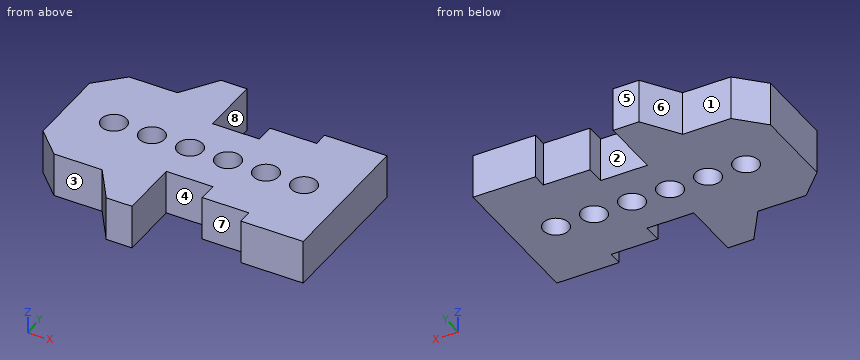
from build123d import *

# Parameters (mm, degrees)
BOSS_EXTRUDE1_DEPTH = 22.225


with BuildPart() as part:
    # Sketch4 → Boss-Extrude1 (new body)
    with BuildSketch(Plane.XY):
        with BuildLine():
            Line((-49.139399536, 0.154397006), (-66.665399536, 0.154397006))
            Line((-66.665399536, 0.154397006), (-66.665399536, -20.419602994))
            Line((-66.665399536, -20.419602994), (-53.965399536, -33.119602994))
            Line((-53.965399536, -33.119602994), (-29.835399536, -33.119602994))
            Line((-29.835399536, -33.119602994), (-17.897399536, -50.645602994))
            Line((-17.897399536, -50.645602994), (-4.943399536, -50.645602994))
            Line((-4.943399536, -50.645602994), (-4.943399536, -20.419602994))
            Line((-4.943399536, -20.419602994), (18.424600464, -20.419602994))
            Line((18.424600464, -20.419602994), (18.424600464, -29.817602994))
            Line((18.424600464, -29.817602994), (41.792600464, -29.817602994))
            Line((41.792600464, -29.817602994), (41.792600464, -36.929602994))
            Line((41.792600464, -36.929602994), (73.034600464, -36.929602994))
            Line((73.034600464, -36.929602994), (73.034600464, 0.154397006))
            Line((73.034600464, 0.154397006), (58.810600464, 0.154397006))
            ThreePointArc((58.810600464, 0.154397006), (52.460600464, -6.195602994), (46.110600464, 0.154397006))
            Line((46.110600464, 0.154397006), (39.760600464, 0.154397006))
            ThreePointArc((39.760600464, 0.154397006), (33.410600464, -6.195602994), (27.060600464, 0.154397006))
            Line((27.060600464, 0.154397006), (20.710600464, 0.154397006))
            ThreePointArc((20.710600464, 0.154397006), (14.360600464, -6.195602994), (8.010600464, 0.154397006))
            Line((8.010600464, 0.154397006), (1.660600464, 0.154397006))
            ThreePointArc((1.660600464, 0.154397006), (-4.689399536, -6.195602994), (-11.039399536, 0.154397006))
            Line((-11.039399536, 0.154397006), (-17.389399536, 0.154397006))
            ThreePointArc((-17.389399536, 0.154397006), (-23.739399536, -6.195602994), (-30.089399536, 0.154397006))
            Line((-30.089399536, 0.154397006), (-36.439399536, 0.154397006))
            ThreePointArc((-36.439399536, 0.154397006), (-42.789399536, -6.195602994), (-49.139399536, 0.154397006))
        make_face()
        with BuildLine():
            Line((-53.965399536, 33.428397006), (-66.665399536, 20.728397006))
            Line((-66.665399536, 20.728397006), (-66.665399536, 0.154397006))
            Line((-66.665399536, 0.154397006), (-49.139399536, 0.154397006))
            ThreePointArc((-49.139399536, 0.154397006), (-42.789399536, 6.504397006), (-36.439399536, 0.154397006))
            Line((-36.439399536, 0.154397006), (-30.089399536, 0.154397006))
            ThreePointArc((-30.089399536, 0.154397006), (-23.739399536, 6.504397006), (-17.389399536, 0.154397006))
            Line((-17.389399536, 0.154397006), (-11.039399536, 0.154397006))
            ThreePointArc((-11.039399536, 0.154397006), (-4.689399536, 6.504397006), (1.660600464, 0.154397006))
            Line((1.660600464, 0.154397006), (8.010600464, 0.154397006))
            ThreePointArc((8.010600464, 0.154397006), (14.360600464, 6.504397006), (20.710600464, 0.154397006))
            Line((20.710600464, 0.154397006), (27.060600464, 0.154397006))
            ThreePointArc((27.060600464, 0.154397006), (33.410600464, 6.504397006), (39.760600464, 0.154397006))
            Line((39.760600464, 0.154397006), (46.110600464, 0.154397006))
            ThreePointArc((46.110600464, 0.154397006), (52.460600464, 6.504397006), (58.810600464, 0.154397006))
            Line((58.810600464, 0.154397006), (73.034600464, 0.154397006))
            Line((73.034600464, 0.154397006), (73.034600464, 37.238397006))
            Line((73.034600464, 37.238397006), (41.792600464, 37.238397006))
            Line((41.792600464, 37.238397006), (41.792600464, 30.126397006))
            Line((41.792600464, 30.126397006), (18.424600464, 30.126397006))
            Line((18.424600464, 30.126397006), (18.424600464, 20.728397006))
            Line((18.424600464, 20.728397006), (-4.943399536, 20.728397006))
            Line((-4.943399536, 20.728397006), (-4.943399536, 50.954397006))
            Line((-4.943399536, 50.954397006), (-17.897399536, 50.954397006))
            Line((-17.897399536, 50.954397006), (-29.835399536, 33.428397006))
            Line((-29.835399536, 33.428397006), (-53.965399536, 33.428397006))
        make_face()
    extrude(amount=BOSS_EXTRUDE1_DEPTH)


solid = part.part
Build history of the part. All positions in model axes, mm. Face numbers are marked on the shaded views. A direction names the side the tool comes from. Round coordinates to 2 decimals unless told otherwise and drop trailing zeros. Write each loop counter-clockwise with the first axis right and the second up, starting at its lowest first coordinate (ties: lowest second). Pieces come first, ordered by that corner, then holes. Notation, with made-up numbers: M 73.5,73.25 L 125.5,73.25 A27 cw 125.5,89.25 Z; hole C 85.25,-23.5 d6. An arc over 180 degrees is marked long. Answer as a JSON object with one key per item and string values. Group by question number.
(1) Drill centre lines: L1, parallel to Y at x = 63, z = 5; L2, parallel to Y at x = 3.5, z = 13.5; L3, parallel to X at y = 22, z = 3.5. Where is each one in solid material? Low to high.
(2) Mould opens along X. For the marked faces 5, 6, 7 and 8 say: pulls with the +X half, pulls with the -X half, needs draft (parallel to the pull), parting line crosses it, or undercut.
(3) Cut at A-A (x = -2). Give the cut face in (y, z) (3 decimals).
(4) Cut at C-C (x = 44). Give the cut face in (y, z) (3 decimals), and give its area (3 significant figures).
(5) Flat gauge pins, fed straight in: pin 1 (6.5 mm diameter, centred on x = 3.5, z = 15, fed in from -Y); pin 2 (6.5 mm diameter, centred on x = -42.5, z = 11, fed in from +Y); pin 3 (6.5 mm diameter, centred on x = 28, z = 9, fed in from +Y). Where does each tip first touch, or does it go through?
(6) Cut at D-D (y = -42). Give the cut face in (x, z) (3 decimals).
(7) Which spindle directions (+Z, -Z, +X, -X, +Y, -Y) get a long thin tool onto all of the face, cutting with end or side? Do the marked faces 1, 2, 3 and 4. Say none if no direction does.
(8) Cut at B-B (z = 12.5). Give the cut face in (x, y).
Responses:
{
 "1": {"L1": "y = -36.93 to 37.24", "L2": "y = -20.42 to 20.73", "L3": "x = -65.39 to -4.94, 18.42 to 73.03"},
 "2": {"face 5": "needs draft", "face 6": "pulls with the -X half", "face 7": "undercut", "face 8": "undercut"},
 "3": {"outline": "M -20.42,0 L -5.598,0 L -5.598,22.225 L -20.42,22.225 Z; M 5.907,0 L 20.728,0 L 20.728,22.225 L 5.907,22.225 Z"},
 "4": {"outline": "M -36.93,0 L 37.238,0 L 37.238,22.225 L -36.93,22.225 Z", "area": "1,650 mm2"},
 "5": {"pin 1": "stops at y = -20.42", "pin 2": "stops at y = 33.43", "pin 3": "stops at y = 30.13"},
 "6": {"outline": "M -23.786,0 L -4.943,0 L -4.943,22.225 L -23.786,22.225 Z"},
 "7": {"face 1": "+Z, -Z, -X, +Y", "face 2": "+Z, -Z, +Y", "face 3": "+Z, -Z, -X, -Y", "face 4": "+Z, -Z, -Y"},
 "8": {"outline": "M -66.67,-20.42 L -53.97,-33.12 L -29.84,-33.12 L -17.9,-50.65 L -4.94,-50.65 L -4.94,-20.42 L 18.42,-20.42 L 18.42,-29.82 L 41.79,-29.82 L 41.79,-36.93 L 73.03,-36.93 L 73.03,37.24 L 41.79,37.24 L 41.79,30.13 L 18.42,30.13 L 18.42,20.73 L -4.94,20.73 L -4.94,50.95 L -17.9,50.95 L -29.84,33.43 L -53.97,33.43 L -66.67,20.73 Z; hole C -42.79,0.15 d12.7; hole C -23.74,0.15 d12.7; hole C -4.69,0.15 d12.7; hole C 14.36,0.15 d12.7; hole C 33.41,0.15 d12.7; hole C 52.46,0.15 d12.7"}
}
